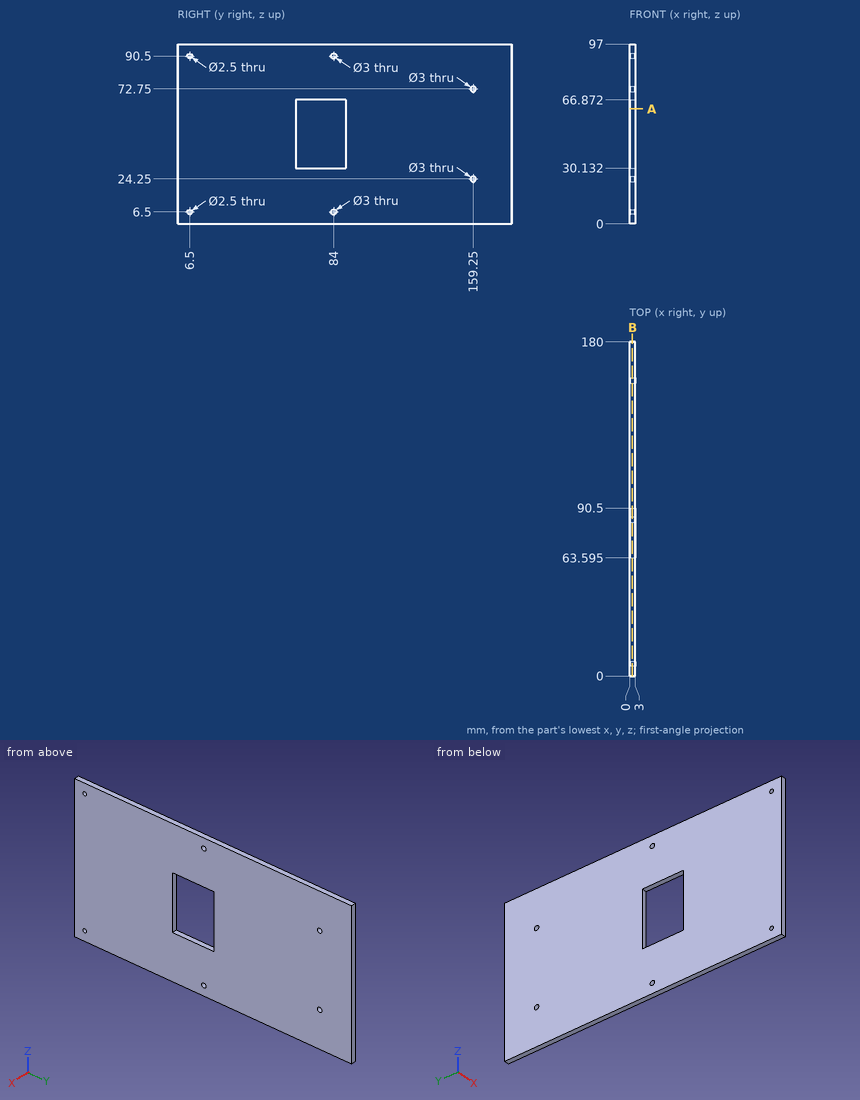
The drawing under review shows one solid part. Ordinate dimensions are in mm from its lowest x, y, z. Coordinates: 2 decimals unless noted, no trailing zeros. Write each loop counter-clockwise with the first axis right and the second up, starting at its lowest first coordinate (ties: lowest second). Pieces come first, ordered by that corner, then holes.
1) Add section A-A (z = 62). Write out the cut boundary in (x, y) (1 decimal), plus the area to 3 significant figures.
2) To check wall thickness, follow L1, parallel to Z at x = 2.1, y = 159.25; L2, parallel to Y at x = 1.95, z = 90.5; L3, parallel to Z at x = 0.75, y = 84. State the ranges of each line that lie inside material, in increasing order.
3) Add section B-B (x = 1.45). State how many separate pieces and enclosed holes the cut face has, plus the area to 3 significant figures.
Check result:
1. outline: (0, 0) - (3, 0) - (3, 63.6) - (0, 63.6) - close; (0, 90.5) - (3, 90.5) - (3, 180) - (0, 180) - close
1. area: 459 mm2
2. L1: z = 0 to 22.75, 25.75 to 71.25, 74.25 to 97
2. L2: y = 0 to 5.25, 7.75 to 82.5, 85.5 to 180
2. L3: z = 0 to 5, 8 to 30.13, 66.87 to 89, 92 to 97
3. separate pieces: 1
3. enclosed holes: 7
3. area: 16,400 mm2
